Work out the finished part from the listing and answer in its coordinate system (mm). Round coordinates to 2 decimals unless told otherwise and drop trailing zeros. Order: outer loops, then holes, each group sorted by start corner. A loop starts at its lowest first (then second) coordinate and runs counter-clockwise, first axis right, second up. Notation, with made-up numbers: (70, -38.75) -> (111, -38.75) arc R13 ccw to (111, -23.75) -> close; hole circle Ø7 at (23.5, 39.25). An arc over 180 degrees is marked (long way). Use one line per item in the form item = value.
```python
from build123d import *

# Parameters (mm, degrees)
CROQUIS1_W              = 40
CROQUIS1_H              = 40
CROQUIS1_W_2            = 39
CROQUIS1_H_2            = 39
SALIENTE_EXTRUIR2_DEPTH = 600
CORTAR_EXTRUIR2_DEPTH   = 600
CORTAR_EXTRUIR1_DEPTH   = 600
CROQUIS7_R              = 8
CORTAR_EXTRUIR3_DEPTH   = 550
CROQUIS8_R              = 8
CORTAR_EXTRUIR4_DEPTH   = 550
CROQUIS9_R              = 1.5
CORTAR_EXTRUIR5_DEPTH   = 550
CROQUIS10_R             = 1.5
CORTAR_EXTRUIR6_DEPTH   = 550


with BuildPart() as part:
    # Croquis1 → Saliente-Extruir2 (new body)
    with BuildSketch(Plane.XY):
        Rectangle(CROQUIS1_W, CROQUIS1_H)
        Rectangle(CROQUIS1_W_2, CROQUIS1_H_2, mode=Mode.SUBTRACT)
    extrude(amount=SALIENTE_EXTRUIR2_DEPTH)

    # Croquis6 → Cortar-Extruir2 (cut)
    with BuildSketch(Plane(origin=(0, 20, 0), x_dir=(1, 0, 0), z_dir=(0, 1, 0))):
        Polygon((20, -600), (-20, -560), (-20, -600), align=None)
    extrude(amount=-CORTAR_EXTRUIR2_DEPTH, mode=Mode.SUBTRACT)

    # Croquis5 → Cortar-Extruir1 (cut)
    with BuildSketch(Plane(origin=(0, 20, 0), x_dir=(1, 0, 0), z_dir=(0, 1, 0))):
        Polygon((20, 0), (-20, -40), (-20, 0), align=None)
    extrude(amount=-CORTAR_EXTRUIR1_DEPTH, mode=Mode.SUBTRACT)

    # Croquis7 → Cortar-Extruir3 (cut)
    with BuildSketch(Plane(origin=(20, 0, 0), x_dir=(0, 0, -1), z_dir=(1, 0, 0))):
        with Locations(Location((-540, 0, 0), (0, 0, 90))):
            Circle(CROQUIS7_R)
    extrude(amount=-CORTAR_EXTRUIR3_DEPTH, mode=Mode.SUBTRACT)

    # Croquis8 → Cortar-Extruir4 (cut)
    with BuildSketch(Plane(origin=(20, 0, 0), x_dir=(0, 0, -1), z_dir=(1, 0, 0))):
        with Locations(Location((-60, 0, 0), (0, 0, 90))):
            Circle(CROQUIS8_R)
    extrude(amount=-CORTAR_EXTRUIR4_DEPTH, mode=Mode.SUBTRACT)

    # Croquis9 → Cortar-Extruir5 (cut)
    with BuildSketch(Plane(origin=(0, 20, 0), x_dir=(1, 0, 0), z_dir=(0, 1, 0))):
        with Locations(Location((0, -562.380435737, 0), (0, 0, 270))):
            Circle(CROQUIS9_R)
        with Locations(Location((0, -462.380435737, 0), (0, 0, 270))):
            Circle(CROQUIS9_R)
        with Locations(Location((0, -362.380435737, 0), (0, 0, 270))):
            Circle(CROQUIS9_R)
        with Locations(Location((0, -262.380435737, 0), (0, 0, 270))):
            Circle(CROQUIS9_R)
        with Locations(Location((0, -162.380435737, 0), (0, 0, 270))):
            Circle(CROQUIS9_R)
        with Locations(Location((0, -72.380435737, 0), (0, 0, 270))):
            Circle(CROQUIS9_R)
    extrude(amount=-CORTAR_EXTRUIR5_DEPTH, mode=Mode.SUBTRACT)

    # Croquis10 → Cortar-Extruir6 (cut)
    with BuildSketch(Plane(origin=(20, 0, 0), x_dir=(0, 0, -1), z_dir=(1, 0, 0))):
        with Locations(Location((-200, 17, 0), (0, 0, 90))):
            Circle(CROQUIS10_R)
        with Locations(Location((-231, 17, 0), (0, 0, 90))):
            Circle(CROQUIS10_R)
        with Locations(Location((-200, -14, 0), (0, 0, 90))):
            Circle(CROQUIS10_R)
        with Locations(Location((-231, -14, 0), (0, 0, 90))):
            Circle(CROQUIS10_R)
        with Locations(Location((-369, 17, 0), (0, 0, 90))):
            Circle(CROQUIS10_R)
        with Locations(Location((-400, 17, 0), (0, 0, 90))):
            Circle(CROQUIS10_R)
        with Locations(Location((-369, -14, 0), (0, 0, 90))):
            Circle(CROQUIS10_R)
        with Locations(Location((-400, -14, 0), (0, 0, 90))):
            Circle(CROQUIS10_R)
    extrude(amount=-CORTAR_EXTRUIR6_DEPTH, mode=Mode.SUBTRACT)


solid = part.part
```
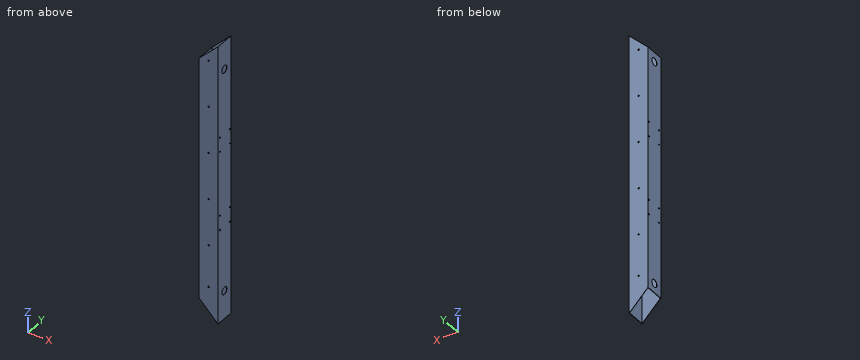
Item 1: The part is cut by section A-A, the plane y = 0. Give the vertices of the cut face in (x, z), and give its area (3 significant figures).
Findings:
outline = (-20, 40) -> (-19.5, 39.5) -> (-19.5, 52) -> (-20, 52) -> close; (-20, 68) -> (-19.5, 68) -> (-19.5, 532) -> (-20, 532) -> close; (-20, 548) -> (-19.5, 548) -> (-19.5, 560.5) -> (-20, 560) -> close; (19.5, 0.5) -> (20, 0) -> (20, 52) -> (19.5, 52) -> close; (19.5, 68) -> (20, 68) -> (20, 532) -> (19.5, 532) -> close; (19.5, 548) -> (20, 548) -> (20, 600) -> (19.5, 599.5) -> close
area = 528 mm^2
Item 2: Consider line 1 along X through (y, z) = (15.5, 83); line 2 along Z through (x, y) = (19.6, 17). Determine where each line is inside the solid, lowest interval first.
Findings:
line_1 = -20 to -19.5, 19.5 to 20
line_2 = 0.4 to 198.5, 201.5 to 229.5, 232.5 to 367.5, 370.5 to 398.5, 401.5 to 599.6
Item 3: The part is cut by section C-C, the plane z = 355. Give the vertices of the cut face in (x, y).
Findings:
outline = (-20, -20) -> (20, -20) -> (20, 20) -> (-20, 20) -> close; hole (-19.5, -19.5) -> (19.5, -19.5) -> (19.5, 19.5) -> (-19.5, 19.5) -> close
Item 4: A flat-ended cylindrical pin translates along its axis: P1, Ø3.5, axis at y = -14, z = 231, coming from the -X side. Find the tip coordinate at first contact, or state that the pin passes through.
Findings:
P1 = -20
Item 5: The part is cut by section B-B, the plane x = -11.5. Give the vertices of the cut face in (y, z), and give its area (3 significant figures).
Findings:
outline = (-20, 31.5) -> (-19.5, 31.5) -> (-19.5, 568.5) -> (-20, 568.5) -> close; (19.5, 31.5) -> (20, 31.5) -> (20, 568.5) -> (19.5, 568.5) -> close
area = 537 mm^2
Item 6: The part is cut by section D-D, the plane z = 60. Give the vertices of the cut face in (x, y).
Findings:
outline = (-20, -20) -> (20, -20) -> (20, -8) -> (19.5, -8) -> (19.5, -19.5) -> (-19.5, -19.5) -> (-19.5, -8) -> (-20, -8) -> close; (-20, 8) -> (-19.5, 8) -> (-19.5, 19.5) -> (19.5, 19.5) -> (19.5, 8) -> (20, 8) -> (20, 20) -> (-20, 20) -> close
